CAD build for the part. Positions are in the model's coordinates, mm. Face numbers are marked on the shaded views. A direction names the side the tool comes from. Round coordinates to 2 decimals unless told otherwise and drop trailing zeros. Write each loop counter-clockwise with the first axis right and the second up, starting at its lowest first coordinate (ties: lowest second). Pieces come first, ordered by that corner, then holes. Notation, with made-up numbers: (34, -23.75) -> (58, -23.75) arc R21 ccw to (58, -15.75) -> close; hole circle Ø8 at (27.5, 39.25). An arc over 180 degrees is marked (long way). Put each result on its own line as item: value. Start each with the question number.
1. Drill centre lines: line 1 (Y direction, x = 5.25, z = 5.75); line 2 (X direction, y = 1.85, z = 4); line 3 (Z direction, x = 4, y = 19.9). Where is each one in solid material? Low to high. Write a range as from..to.
2. Saw through at C-C on x = 4. List the corners of the cut face in (y, z).
3. Saw through at A-A on z = 4. List the corners of the cut face in (x, y).
4. Saw through at B-B on z = 6.25. List the corners of the cut face in (x, y), and give its area (3 significant figures).
5. Flat gauge pins, fed straight in: P1, Ø1.5, axis at y = 5, z = 9, coming from the -X side; P2, Ø2, axis at x = 4, z = 4, coming from the -Y side; P3, Ø4, axis at x = 4, y = 13.5, coming from the -Z side. Where does each tip first touch, or does it go through?
6. Pull direction X, two halves, no side cores. Call the marked faces 1, 2 and 3: pulls with the +X half, pulls with the -X half, needs draft (parallel to the pull), parting line crosses it, or undercut.
7. 3-axis set-ups, long thin cutter, end or side, ignore diameter. For the marked faces 4 and 5: which of +Z, -Z, +X, -X, +Y, -Y reach the whole face in a straight line?
8. Saw through at D-D on y = 16.5. List the corners of the cut face in (x, z), and give its area (3 significant figures).
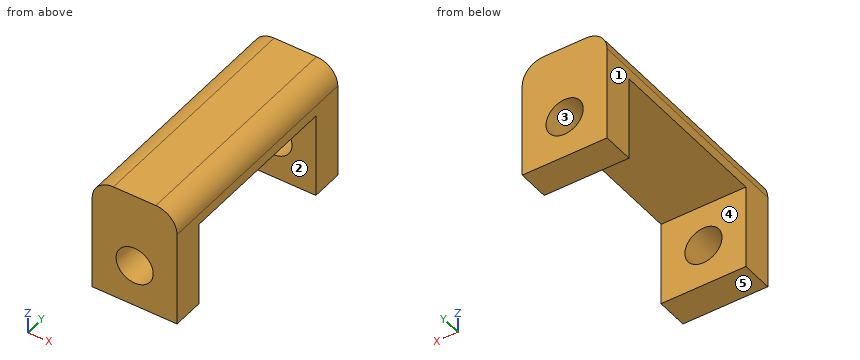
from build123d import *

# Parameters (mm, degrees)
SKETCH_1_W      = 8
SKETCH_1_H      = 8
SKETCH_1_R      = 1.75
EXTRUDE_1_DEPTH = 3
EXTRUDE_2_DEPTH = 16
SKETCH_3_R      = 1.75
EXTRUDE_3_DEPTH = 3


with BuildPart() as part:
    # 草图1 → 凸台-拉伸1 (new body)
    with BuildSketch(Plane(origin=(0, 0, 0), x_dir=(1, 0, 0), z_dir=(0, 1, 0))):
        with Locations((4, -4)):
            Rectangle(SKETCH_1_W, SKETCH_1_H)
        with Locations((4, -4)):
            Circle(SKETCH_1_R, mode=Mode.SUBTRACT)
        with BuildLine():
            Line((8, -8), (0, -8))
            Line((0, -8), (0, -9))
            ThreePointArc((0, -9), (0.585786438, -10.414213562), (2, -11))
            Line((2, -11), (6, -11))
            ThreePointArc((6, -11), (7.414213562, -10.414213562), (8, -9))
            Line((8, -9), (8, -8))
        make_face()
    extrude(amount=EXTRUDE_1_DEPTH)

    # 草图2 → 凸台-拉伸2 (add)
    with BuildSketch(Plane(origin=(0, 3, 0), x_dir=(1, 0, 0), z_dir=(0, 1, 0))):
        with BuildLine():
            Line((8, -8), (0, -8))
            Line((0, -8), (0, -9))
            ThreePointArc((0, -9), (0.585786438, -10.414213562), (2, -11))
            Line((2, -11), (6, -11))
            ThreePointArc((6, -11), (7.414213562, -10.414213562), (8, -9))
            Line((8, -9), (8, -8))
        make_face()
    extrude(amount=EXTRUDE_2_DEPTH)

    # 草图3 → 凸台-拉伸3 (add)
    with BuildSketch(Plane(origin=(0, 19, 0), x_dir=(1, 0, 0), z_dir=(0, 1, 0))):
        with BuildLine():
            Line((8, -9), (8, -8))
            Line((8, -8), (8, 0))
            Line((8, 0), (0, 0))
            Line((0, 0), (0, -8))
            Line((0, -8), (0, -9))
            ThreePointArc((0, -9), (0.585786438, -10.414213562), (2, -11))
            Line((2, -11), (6, -11))
            ThreePointArc((6, -11), (7.414213562, -10.414213562), (8, -9))
        make_face()
        with Locations((4, -4)):
            Circle(SKETCH_3_R, mode=Mode.SUBTRACT)
    extrude(amount=EXTRUDE_3_DEPTH)


solid = part.part
Return value:
1. line 1: y = 0..3, 19..22
1. line 2: x = 0..2.25, 5.75..8
1. line 3: z = 0..2.25, 5.75..11
2. outline: (0, 0) -> (3, 0) -> (3, 2.25) -> (0, 2.25) -> close; (0, 5.75) -> (3, 5.75) -> (3, 8) -> (19, 8) -> (19, 5.75) -> (22, 5.75) -> (22, 11) -> (0, 11) -> close; (19, 0) -> (22, 0) -> (22, 2.25) -> (19, 2.25) -> close
3. outline: (0, 0) -> (2.25, 0) -> (2.25, 3) -> (0, 3) -> close; (0, 19) -> (2.25, 19) -> (2.25, 22) -> (0, 22) -> close; (5.75, 0) -> (8, 0) -> (8, 3) -> (5.75, 3) -> close; (5.75, 19) -> (8, 19) -> (8, 22) -> (5.75, 22) -> close
4. outline: (0, 0) -> (8, 0) -> (8, 3) -> (0, 3) -> close; (0, 19) -> (8, 19) -> (8, 22) -> (0, 22) -> close
4. area: 48.0 mm^2
5. P1: stops at x = 0
5. P2: passes through
5. P3: stops at z = 8
6. face 1: pulls with the -X half
6. face 2: needs draft
6. face 3: undercut
7. face 4: -Z, +X, -X
7. face 5: -Z, +X, -X, +Y, -Y
8. outline: (0, 8) -> (8, 8) -> (8, 9) arc R2 ccw to (6, 11) -> (2, 11) arc R2 ccw to (0, 9) -> close
8. area: 22.3 mm^2
